```python
from build123d import *

# Parameters (mm, degrees)
EXTRUDE_1_DEPTH        = 24.5
SHELL_1_T              = -2
CUT_EXTRUDE_1_DEPTH    = 365.204612821
HOLE_WIZARD_M4_1_D     = 4.5
HOLE_WIZARD_M4_2_D     = 4.5
HOLE_WIZARD_M4_2_DEPTH = 2


with BuildPart() as part:
    # 草图1 → 拉伸-薄壁1 (new, symmetric)
    with BuildSketch(Plane.XY):
        with BuildLine():
            Line((12, 0), (12, 300))
            ThreePointArc((12, 300), (38, 326), (64, 300))
            Line((64, 300), (64, 238))
            Line((64, 238), (88, 238))
            Line((88, 238), (88, 300))
            ThreePointArc((88, 300), (38, 350), (-12, 300))
            Line((-12, 300), (-12, 0))
            Line((-12, 0), (12, 0))
        make_face()
    extrude(amount=EXTRUDE_1_DEPTH, both=True)

    # 抽壳1
    shell_1_openings = [part.faces().sort_by_distance(p)[0] for p in [
        (0, 0, 0),
        (76, 238, 0),
    ]]
    offset(amount=SHELL_1_T, openings=shell_1_openings, kind=Kind.INTERSECTION)

    # 草图2 → 切除-拉伸1 (cut, through all)
    with BuildSketch(Plane.XY.offset(24.5)):
        Polygon((88, 263), (88, 238), (72, 238), align=None)
        Polygon((12, 25), (12, 0), (-4, 0), align=None)
    extrude(amount=-CUT_EXTRUDE_1_DEPTH, mode=Mode.SUBTRACT)

    # M4 间隙孔1 (through all)
    with Locations(Plane(origin=(-10, 0, 0), x_dir=(0, 0, -1), z_dir=(1, 0, 0))):
        with Locations((12.5, 10), (-12.5, 10)):
            Hole(HOLE_WIZARD_M4_1_D / 2)

    # M4 间隙孔2
    with Locations(Plane(origin=(66, 0, 0), x_dir=(0, 0, -1), z_dir=(1, 0, 0))):
        with Locations((12.5, 248), (-12.5, 248)):
            Hole(HOLE_WIZARD_M4_2_D / 2, depth=HOLE_WIZARD_M4_2_DEPTH)


solid = part.part
```
Check sheet for the modelled part. Datum: model origin and axes. Units: mm. A direction names the side the tool comes from. Round coordinates to 2 decimals unless told otherwise and drop trailing zeros. Write each loop counter-clockwise with the first axis right and the second up, starting at its lowest first coordinate (ties: lowest second). Pieces come first, ordered by that corner, then holes. Notation, with made-up numbers: (65, 88) -> (123, 88) arc R19 cw to (123, 93) -> close; hole circle Ø11 at (-20, -1). An arc over 180 degrees is marked (long way). Put each result on its own line as item: value.
(1) Sectioned sample at A-A (y = 256). Enter the section's corners in (x, z), plus the area to 3 significant figures.
Values found:
outline: (-12, -24.5) -> (12, -24.5) -> (12, 24.5) -> (-12, 24.5) -> close; (64, -24.5) -> (83.52, -24.5) -> (83.52, -22.5) -> (66, -22.5) -> (66, 22.5) -> (83.52, 22.5) -> (83.52, 24.5) -> (64, 24.5) -> close; hole (-10, -22.5) -> (10, -22.5) -> (10, 22.5) -> (-10, 22.5) -> close
area: 444 mm^2
(2) Tool access check on faces 1 (the face through (12, 161, 0)), 2 (the face through (65.6, 238, 0.1)), 3 (the face through (-10, 152, 0)), 4 (the face through (9, 213, -22.5)). Record the directions out of +Z, -Z, +X, -X, +Y, -Y that give a thin tool (end or side, any length) a straight path to the whole face; none if there is none.
Values found:
face 1: +Z, -Z, -Y
face 2: +Z, -Z, +X, -Y
face 3: -Y
face 4: none
(3) Sectioned sample at C-C (z = 18). Enter the section's corners in (x, y) (3 decimals), plus the area to 3 significant figures.
Values found:
outline: (-12, 0) -> (-10, 0) -> (-10, 300) arc R48 cw to (86, 300) -> (86, 259.875) -> (88, 263) -> (88, 300) arc R50 ccw to (-12, 300) -> close; (10, 21.875) -> (12, 25) -> (12, 300) arc R26 cw to (64, 300) -> (64, 238) -> (66, 238) -> (66, 300) arc R28 ccw to (10, 300) -> close
area: 1,830 mm^2
(4) Mould release check, pull along X, two halves, no side actions. Record for faces 5 (the face through (11.8, 214.7, -24.5)), 6 (the face through (39.06, 347.99, 0.32)), 7 (the face through (-12, 152, 0)), 8 (the face through (88, 281, 0)): released by +X, released by -X, zero draft, split by the parting line, or undercut.
Values found:
face 5: zero draft
face 6: undercut
face 7: released by -X
face 8: released by +X
(5) Sectioned sample at B-B (x = 38). Enter the section's corners in (y, z), plus the area to 3 significant figures.
Values found:
outline: (326, -24.5) -> (350, -24.5) -> (350, 24.5) -> (326, 24.5) -> close; hole (328, -22.5) -> (348, -22.5) -> (348, 22.5) -> (328, 22.5) -> close
area: 276 mm^2
(6) Sectioned sample at D-D (y = 185). Enter the section's corners in (x, z), plus the area to 3 significant figures.
Values found:
outline: (-12, -24.5) -> (12, -24.5) -> (12, 24.5) -> (-12, 24.5) -> close; hole (-10, -22.5) -> (10, -22.5) -> (10, 22.5) -> (-10, 22.5) -> close
area: 276 mm^2
(7) Material ranges on line 1 (X direction, y = 283, z = 17); line 2 (Z direction, x = 64.85, y = 248); line 3 (X direction, y = 256, z = -5.5), recorded low to high.
Values found:
line 1: x = -12 to -10, 10 to 12, 64 to 66, 86 to 88
line 2: z = -24.5 to -14.75, -10.25 to 10.25, 14.75 to 24.5
line 3: x = -12 to -10, 10 to 12, 64 to 66
(8) Go/stop test with flat-tipped pins: pin 1 Ø2.5 at (y, z) = (10, 12.5) entering from -X; pin 2 Ø1 at (y, z) = (127.5, 9) entering from +X; pin 3 Ø8 at (x, z) = (61, -14.5) entering from -Y; pin 4 Ø5 at (y, z) = (248, -12.5) entering from +X. Record where each tip stops, or that it passes through.
Values found:
pin 1: passes through
pin 2: stops at x = 12
pin 3: stops at y = 238
pin 4: stops at x = 66
